Work out the finished part from the listing and answer in its coordinate system (mm). Face numbers are marked on the shaded views. A direction names the side the tool comes from. Round coordinates to 2 decimals unless told otherwise and drop trailing zeros. Loops run counter-clockwise (first coordinate to the right, second up) from the corner with the lowest first, then second, coordinate; pieces in that order, holes last.
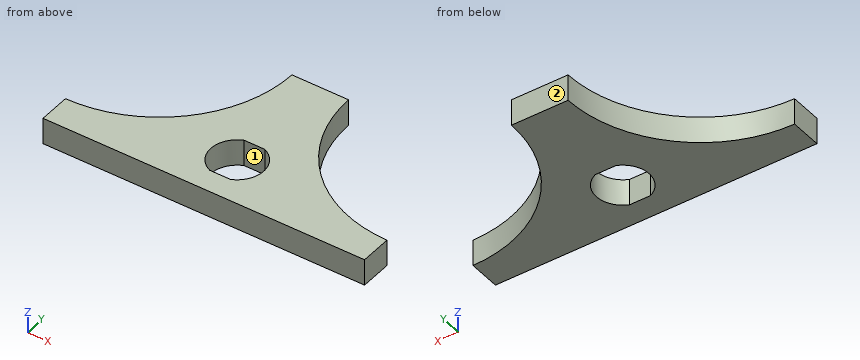
```python
from build123d import *

# Parameters (mm, degrees)
SKETCH1_W           = 129.563097232
SKETCH1_H           = 81.098705598
BOSS_EXTRUDE1_DEPTH = 6.35
SKETCH2_R           = 6.35
CUT_EXTRUDE1_DEPTH  = 77.689122785
SKETCH4_OUTSIDE_W   = 162.16
SKETCH4_OUTSIDE_H   = 113.694
CUT_EXTRUDE2_DEPTH  = 77.689122785
SKETCH6_W           = 4.977363158
SKETCH6_H           = 1.27
BOSS_EXTRUDE2_DEPTH = 6.35


with BuildPart() as part:
    # Sketch1 → Boss-Extrude1 (new body)
    with BuildSketch(Plane.XY):
        Rectangle(SKETCH1_W, SKETCH1_H)
    extrude(amount=BOSS_EXTRUDE1_DEPTH)

    # Sketch2 → Cut-Extrude1 (cut, through all)
    with BuildSketch(Plane.XY.offset(6.35)):
        Circle(SKETCH2_R)
    extrude(amount=-CUT_EXTRUDE1_DEPTH, mode=Mode.SUBTRACT)

    # Sketch4 outside → Cut-Extrude2 (cut, through all)
    with BuildSketch(Plane.XY.offset(6.35)):
        Rectangle(SKETCH4_OUTSIDE_W, SKETCH4_OUTSIDE_H)
        with BuildLine():
            Line((-38.735, -11.358813087), (38.735, -11.358813087))
            Line((38.735, -11.358813087), (38.735, -3.738813087))
            ThreePointArc((38.735, -3.738813087), (16.172106496, 5.607043409), (6.82625, 28.169936913))
            Line((6.82625, 28.169936913), (-6.82625, 28.169936913))
            ThreePointArc((-6.82625, 28.169936913), (-16.172106496, 5.607043409), (-38.735, -3.738813087))
            Line((-38.735, -3.738813087), (-38.735, -11.358813087))
        make_face(mode=Mode.SUBTRACT)
    extrude(amount=-CUT_EXTRUDE2_DEPTH, mode=Mode.SUBTRACT)

    # Sketch6 → Boss-Extrude2 (add)
    with BuildSketch(Plane.XY.offset(6.35)):
        with Locations((0, 6.477)):
            Rectangle(SKETCH6_W, SKETCH6_H)
    boss_extrude2 = extrude(amount=-BOSS_EXTRUDE2_DEPTH)

    # Mirror1: Boss-Extrude2 across plane
    add(boss_extrude2.mirror(Plane.ZX))


solid = part.part
```
1. Given pin 1 (3 mm diameter, centred on y = 1, z = 0.5, fed in from +X); pin 2 (10 mm diameter, centred on x = -30.5, y = 4.5, fed in from +Z), each flat-ended and moving along its own axis, determine where each tip first touches the part or whether it passes through.
Answer key:
pin 1: stops at x = 24.73
pin 2: passes through
2. Which of the six approach directions +Z, -Z, +X, -X, +Y, -Y give full straight-line access (tool end or side, diameter ignored) to the marked faces 1 and 2?
Answer key:
face 1: +Z, -Z
face 2: +Z, -Z, +X, -X, +Y
3. Find section B-B (x = -26). Write down the section's boundary in (y, z).
Answer key:
outline: (-11.36, 0) - (-1.09, 0) - (-1.09, 6.35) - (-11.36, 6.35) - close
4. Find section C-C (y = 14). Write down the section's boundary in (x, z), then the cut area to 3 significant figures.
Answer key:
outline: (-10.15, 0) - (10.15, 0) - (10.15, 6.35) - (-10.15, 6.35) - close
area: 129 mm2
5. Consider probe 1 along Y at (x, z) = (1.5, 1.25); probe 2 along X at (y, z) = (4.5, 5.5); probe 3 along X at (y, z) = (1, 0.75). Determine where each line is inside the solid, lowest interval first.
Answer key:
probe 1: y = -11.36 to -5.84, 5.84 to 28.17
probe 2: x = -17.34 to -4.48, 4.48 to 17.34
probe 3: x = -22 to -6.27, 6.27 to 22
